Design review of the part built by this model. Coordinates are the model's own, in mm. Face numbers are marked on the shaded views. A direction names the side the tool comes from. Coordinates: 2 decimals unless noted, no trailing zeros. Write each loop counter-clockwise with the first axis right and the second up, starting at its lowest first coordinate (ties: lowest second). Pieces come first, ordered by that corner, then holes. Notation, with made-up numbers: (83.5, 6.5) - (121.5, 6.5) arc R4 cw to (121.5, 11.5) - close; hole circle Ø7 at (74, -12). An arc over 180 degrees is marked (long way). Answer as a JSON object with one key per item and string values.
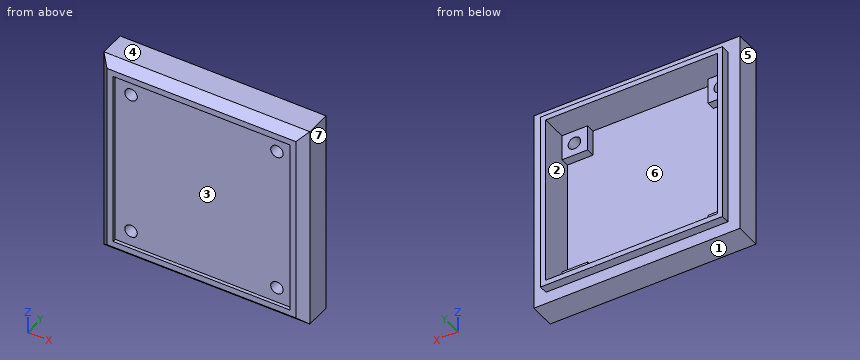
```python
from build123d import *

# Parameters (mm, degrees)
SKETCH1_W               = 120
SKETCH1_H               = 120
SKETCH1_W_2             = 106
SKETCH1_H_2             = 106
BOSS_EXTRUDE1_DEPTH     = 20
SKETCH1_4_W             = 106
SKETCH1_4_H             = 106
SKETCH1_4_W_2           = 100
SKETCH1_4_H_2           = 100
BOSS_EXTRUDE2_DEPTH     = 25
SKETCH1_5_W             = 100
SKETCH1_5_H             = 100
BOSS_EXTRUDE3_DEPTH     = 5
SKETCH1_7_W             = 103
SKETCH1_7_H             = 103
CUT_EXTRUDE1_DEPTH      = 2
SKETCH2_W               = 15
SKETCH2_H               = 15
BOSS_EXTRUDE5_DEPTH     = 5
CUT_EXTRUDE7_DEPTH      = 112
CUT_EXTRUDE7_DEPTH_BACK = 130.755311173
SKETCH8_R               = 3.643912303
CHAMFER1_SIZE           = 5


with BuildPart() as part:
    # Sketch1 → Boss-Extrude1 (new body)
    with BuildSketch(Plane(origin=(0, 0, 0), x_dir=(1, 0, 0), z_dir=(0, 1, 0))):
        with Locations((33.717730969, -27.483870968)):
            Rectangle(SKETCH1_W, SKETCH1_H)
        with Locations((33.717730969, -27.483870968)):
            Rectangle(SKETCH1_W_2, SKETCH1_H_2, mode=Mode.SUBTRACT)
    extrude(amount=BOSS_EXTRUDE1_DEPTH)

    # Sketch1_4 → Boss-Extrude2 (add)
    with BuildSketch(Plane(origin=(0, 0, 0), x_dir=(1, 0, 0), z_dir=(0, 1, 0))):
        with Locations((33.717730969, -27.483870968)):
            Rectangle(SKETCH1_4_W, SKETCH1_4_H)
        with Locations((33.717730969, -27.483870968)):
            Rectangle(SKETCH1_4_W_2, SKETCH1_4_H_2, mode=Mode.SUBTRACT)
    extrude(amount=BOSS_EXTRUDE2_DEPTH)

    # Sketch1_5 → Boss-Extrude3 (add)
    with BuildSketch(Plane(origin=(0, 0, 0), x_dir=(1, 0, 0), z_dir=(0, 1, 0))):
        with Locations((33.717730969, -27.483870968)):
            Rectangle(SKETCH1_5_W, SKETCH1_5_H)
    extrude(amount=BOSS_EXTRUDE3_DEPTH)

    # Sketch1_7 → Cut-Extrude1 (cut)
    with BuildSketch(Plane(origin=(0, 0, 0), x_dir=(1, 0, 0), z_dir=(0, 1, 0))):
        with Locations((33.717730969, -27.483870968)):
            Rectangle(SKETCH1_7_W, SKETCH1_7_H)
    extrude(amount=CUT_EXTRUDE1_DEPTH, mode=Mode.SUBTRACT)

    # Sketch2 → Boss-Extrude5 (add)
    with BuildSketch(Plane(origin=(0, 5, 0), x_dir=(1, 0, 0), z_dir=(0, 1, 0))):
        with Locations((76.217730969, 15.016129032)):
            Rectangle(SKETCH2_W, SKETCH2_H)
        with Locations((-8.782269031, 15.016129032)):
            Rectangle(SKETCH2_W, SKETCH2_H)
        with Locations((-8.782269031, -69.983870968)):
            Rectangle(SKETCH2_W, SKETCH2_H)
        with Locations((76.217730969, -69.983870968)):
            Rectangle(SKETCH2_W, SKETCH2_H)
    extrude(amount=BOSS_EXTRUDE5_DEPTH)

    # Sketch8 → Cut-Extrude7 (cut, two sides: drawn at the far end of the back side and taken through both)
    with BuildSketch(Plane(origin=(0, 5, 0), x_dir=(1, 0, 0), z_dir=(0, 1, 0)).offset(-CUT_EXTRUDE7_DEPTH_BACK)):
        with Locations(Location((-8.562175079, 15.090544671, 0), (0, 0, 90))):
            Circle(SKETCH8_R)
        with Locations(Location((76.437824921, 15.090544671, 0), (0, 0, 90))):
            Circle(SKETCH8_R)
        with Locations(Location((-8.562175079, -69.909455329, 0), (0, 0, 90))):
            Circle(SKETCH8_R)
        with Locations(Location((76.437824921, -69.909455329, 0), (0, 0, 90))):
            Circle(SKETCH8_R)
    extrude(amount=CUT_EXTRUDE7_DEPTH + CUT_EXTRUDE7_DEPTH_BACK, mode=Mode.SUBTRACT)

    # Chamfer1
    chamfer1_edges = [part.edges().sort_by_distance(p)[0] for p in [
        (33.717730969, 0, 87.483870968),
        (-26.282269031, 0, 27.483870968),
        (33.717730969, 0, -32.516129032),
        (93.717730969, 0, 27.483870968),
    ]]
    chamfer(chamfer1_edges, length=CHAMFER1_SIZE)


solid = part.part
```
(1) Tool access review of the marked faces 1, 2 and 3: name each direction out of +Z, -Z, +X, -X, +Y, -Y from which nothing blocks a thin tool from reaching the whole face with its end or side.
Solved:
{"face 1": "-Z, +X, -X, +Y, -Y", "face 2": "+Y", "face 3": "-Y"}
(2) Take a section at B-B, the plane x = 49. Write out the cut boundary in (y, z).
Solved:
{"outline": "(0, -27.52) - (5, -32.52) - (20, -32.52) - (20, -25.52) - (25, -25.52) - (25, -22.52) - (5, -22.52) - (5, 77.48) - (25, 77.48) - (25, 80.48) - (20, 80.48) - (20, 87.48) - (5, 87.48) - (0, 82.48) - (0, 78.98) - (2, 78.98) - (2, -24.02) - (0, -24.02) - close"}
(3) Take a section at A-A, the plane y = 11.5. Write out the cut boundary in (x, z).
Solved:
{"outline": "(-26.28, -32.52) - (93.72, -32.52) - (93.72, 87.48) - (-26.28, 87.48) - close; hole (-16.28, -22.52) - (83.72, -22.52) - (83.72, 77.48) - (-16.28, 77.48) - close"}
(4) Take a section at C-C, the plane z = 24. Write out the cut boundary in (x, y).
Solved:
{"outline": "(-26.28, 5) - (-21.28, 0) - (-17.78, 0) - (-17.78, 2) - (85.22, 2) - (85.22, 0) - (88.72, 0) - (93.72, 5) - (93.72, 20) - (86.72, 20) - (86.72, 25) - (83.72, 25) - (83.72, 5) - (-16.28, 5) - (-16.28, 25) - (-19.28, 25) - (-19.28, 20) - (-26.28, 20) - close"}
(5) For pin 1 (5 mm diameter, centred on x = 18, z = 40.5, fed in from +Y); pin 2 (9.5 mm diameter, centred on x = -8.56, z = 69.91, fed in from +Y); pin 3 (5.5 mm diameter, centred on y = 23.5, z = 47.5, fed in from -X); pin 4 (8 mm diameter, centred on x = 50, y = 3, fed in from +Z), all flat-tipped, find the tip position at first contact; note any pin that passes through.
Solved:
{"pin 1": "stops at y = 5", "pin 2": "stops at y = 10", "pin 3": "stops at x = -19.28", "pin 4": "stops at z = 87.48"}
(6) The part is to be moulded in two halves that separate along X. For the marked faces 4, 5, 6 and 7, say which applies: pulls with the +X half, pulls with the -X half, needs draft (parallel to the pull), parting line crosses it, or undercut.
Solved:
{"face 4": "needs draft", "face 5": "pulls with the -X half", "face 6": "undercut", "face 7": "pulls with the +X half"}
(7) Take a section at D-D, the plane x = 81.5. Write out the cut boundary in (y, z).
Solved:
{"outline": "(0, -27.52) - (5, -32.52) - (20, -32.52) - (20, -25.52) - (25, -25.52) - (25, -22.52) - (10, -22.52) - (10, -7.52) - (5, -7.52) - (5, 62.48) - (10, 62.48) - (10, 77.48) - (25, 77.48) - (25, 80.48) - (20, 80.48) - (20, 87.48) - (5, 87.48) - (0, 82.48) - (0, 78.98) - (2, 78.98) - (2, -24.02) - (0, -24.02) - close"}
(8) To check wall thickness, follow line 1 (X direction, y = 8.25, z = 57); line 2 (Z direction, x = 2.5, y = 17.25); line 3 (Z direction, x = -12.5, y = 22). State the ranges of each line that lie inside material, in increasing order. Write a range as from..to.
Solved:
{"line 1": "x = -26.28..-16.28, 83.72..93.72", "line 2": "z = -32.52..-22.52, 77.48..87.48", "line 3": "z = -25.52..-22.52, 77.48..80.48"}
